Could you check a few things on this drawing? It's one solid part, dimensions in mm from its lowest x, y, z. Give positions to 0.01 mm unless a question says otherwise; leave off trailing zeros.
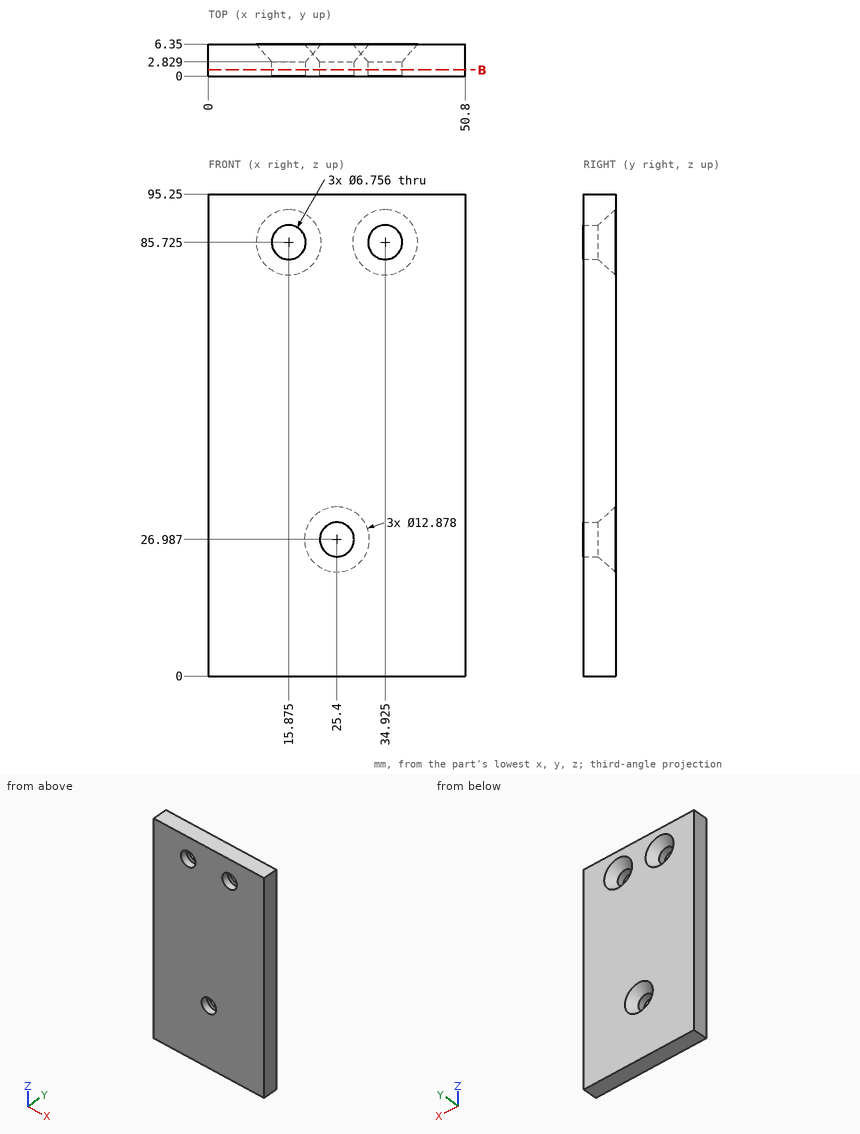
Item 1: For pin 1 (11 mm diameter, centred on x = 25.4, z = 26.99, fed in from +Y) (1 decimal), with a flat end and sliding along its axis, tell me the tip position at first contact or that it passes through.
Findings:
pin 1: stops at y = 5.3
Item 2: Please list where these lines run through material, in increasing order: line 1 along Z through (x, y) = (13, 6.25); line 2 along Z through (x, y) = (17, 1.25); line 3 along X through (y, z) = (2.5, 27.5).
Findings:
line 1: z = 0 to 80.06, 91.39 to 95.25
line 2: z = 0 to 82.54, 88.91 to 95.25
line 3: x = 0 to 22.06, 28.74 to 50.8
Item 3: Imagine slicing it at B-B on y = 1.25. Give the number of separate pieces and of enclosed holes in the cut face, then the cut area to 3 significant figures.
Findings:
separate pieces: 1
enclosed holes: 3
area: 4,730 mm2
